Verification items for the finished model (mm, model axes). Face numbers are marked on the shaded views. Give positions to 0.01 mm unless a question says otherwise; leave off trailing zeros. Write each loop counter-clockwise with the first axis right and the second up, starting at its lowest first coordinate (ties: lowest second). Pieces come first, ordered by that corner, then holes.
from build123d import *

# Parameters (mm, degrees)
ESQUISSE1_R        = 1.25
BOSS_EXTRU_1_DEPTH = 2.4
ESQUISSE2_R        = 2.75
ESQUISSE2_R_2      = 1.25
BOSS_EXTRU_2_DEPTH = 4


with BuildPart() as part:
    # Esquisse1 → Boss.-Extru.1 (new body)
    with BuildSketch(Plane.XY):
        Polygon((3.175426481, 0), (1.58771324, 2.75), (-1.58771324, 2.75), (-3.175426481, 0), (-1.58771324, -2.75), (1.58771324, -2.75), align=None)
        Circle(ESQUISSE1_R, mode=Mode.SUBTRACT)
    extrude(amount=BOSS_EXTRU_1_DEPTH)

    # Esquisse2 → Boss.-Extru.2 (add)
    with BuildSketch(Plane.XY):
        with Locations(Location((0, 0, 0), (0, 0, 150))):
            Circle(ESQUISSE2_R)
        Circle(ESQUISSE2_R_2, mode=Mode.SUBTRACT)
    extrude(amount=BOSS_EXTRU_2_DEPTH)


solid = part.part
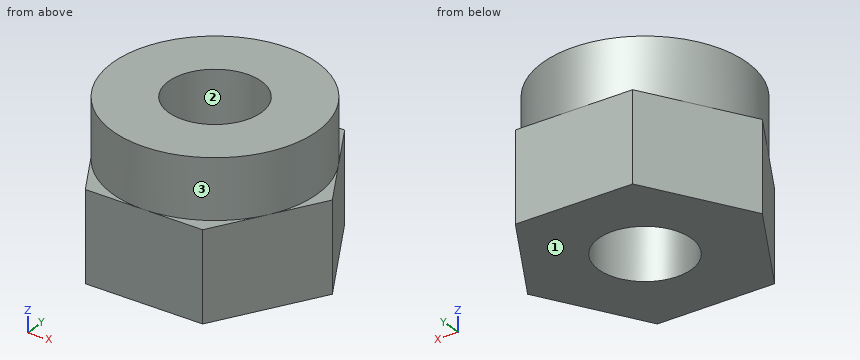
Item 1: Sectioned sample at B-B on y = -0.15. Record the cut outline in (x, z), then the cut area to 3 significant figures.
Answer key:
outline: (-3.09, 0) - (-1.24, 0) - (-1.24, 4) - (-2.75, 4) - (-2.75, 2.4) - (-3.09, 2.4) - close; (1.24, 0) - (3.09, 0) - (3.09, 2.4) - (2.75, 2.4) - (2.75, 4) - (1.24, 4) - close
area: 13.7 mm2
Item 2: Depth check by flat-ended pin: pin 1 (2 mm diameter, centred on y = 1.5, z = 1, fed in from +X); pin 2 (2 mm diameter, centred on x = 2, y = 2, fed in from -Z); pin 3 (1.5 mm diameter, centred on y = 2, z = 2, fed in from +X); pin 4 (2 mm diameter, centred on y = -1.5, z = 3.5, fed in from +X). Enter the tip coordinate at first touch or a pass-through.
Answer key:
pin 1: stops at x = 2.89
pin 2: stops at z = 0
pin 3: stops at x = 2.45
pin 4: stops at x = 2.7
Item 3: Release check for a two-part mould opening along Y. For the marked faces 1, 2 and 3 record: released by +Y, released by -Y, zero draft, split by the parting line, or undercut.
Answer key:
face 1: zero draft
face 2: undercut
face 3: split by the parting line
Item 4: Sectioned sample at A-A on z = 1. Record the cut outline in (x, y).
Answer key:
outline: (-3.18, 0) - (-1.59, -2.75) - (1.59, -2.75) - (3.18, 0) - (1.59, 2.75) - (-1.59, 2.75) - close; hole circle Ø2.5 at (0, 0)
Item 5: Sectioned sample at D-D on y = 2.4. Record the cut outline in (x, z).
Answer key:
outline: (-1.79, 0) - (1.79, 0) - (1.79, 2.4) - (1.34, 2.4) - (1.34, 4) - (-1.34, 4) - (-1.34, 2.4) - (-1.79, 2.4) - close
Item 6: Scan lines: line 1 along Y through (x, z) = (0, 3.85); line 2 along Z through (x, y) = (-1.5, -2.35). Record each from-to range of solid material in increasing order.
Answer key:
line 1: y = -2.75 to -1.25, 1.25 to 2.75
line 2: z = 0 to 2.4
